Autodesk Inventor part; units mm, degrees
ref_plane "YZ Plane" through (0, 0, 0) normal (1, 0, 0) x (0, 1, 0)
ref_plane "XZ Plane" through (0, 0, 0) normal (0, 1, 0) x (-1, 0, 0)
ref_plane "XY Plane" through (0, 0, 0) normal (0, 0, 1) x (1, 0, 0)
sketch "Sketch1" plane through (0, 0, 0) normal (0, 0, 1) x (1, 0, 0)
  line L0 (0, 0) -> (40.6, 0)
  line L1 (40.6, 0) -> (40.6, 36)
  line L2 (40.6, 36) -> (0, 36)
  line L3 (0, 36) -> (0, 0)
  line L4 (0, 29) -> (-7.5, 29)
  line L5 (-7.5, 29) -> (-7.5, 26.5)
  line L6 (-7.5, 26.5) -> (0, 26.5)
  line L7 (0, 26.5) -> (0, 29)
  line L8 (40.6, 29) -> (48.1, 29)
  line L9 (48.1, 29) -> (48.1, 26.5)
  line L10 (48.1, 26.5) -> (40.6, 26.5)
  line L11 (40.6, 26.5) -> (40.6, 29)
  line L12 (0, 5) -> (-3, 5)
  line L13 (-3, 5) -> (-3, 1)
  line L14 (-3, 1) -> (0, 1)
  line L15 (0, 1) -> (0, 5)
  dimension "d0" = 40.6
  dimension "d1" = 36
  dimension "d2" = 7.5
  dimension "d3" = 2.5
  dimension "d4" = 7
  dimension "d5" = 3
  dimension "d6" = 4
  dimension "d7" = 1
extrude "Extrusion1" add sketch "Sketch1" along normal mid plane 20.3 contours L3 L2 L1 L0
extrude "Extrusion2" add sketch "Sketch1" along normal mid plane 18 contours L1 L8 L9 L10 | L6 L5 L4 L3
extrude "Extrusion3" add sketch "Sketch1" along normal mid plane 6 contours L14 L13 L12 L3
sketch "Sketch2" plane through (-7.5, 29, 9) normal (0, 1, 0) x (1, 0, 0)
  line L0 (0, 18) -> (0, 0)
  line L1 (7.5, 18) -> (7.5, 0)
  line L2 (48.1, 0) -> (48.1, 18)
  line L3 (55.6, 0) -> (48.1, 0)
  line L4 (55.6, 18) -> (55.6, 0)
  line L5 (48.1, 18) -> (55.6, 18)
  line L6 (3.5, 14) -> (3.5, 4) construction
  line L7 (0, 9) -> (55.6, 9) construction
  line L8 (52.1, 14) -> (52.1, 4) construction
  line L9 (3.5, 4) -> (52.1, 4) construction
  line L10 (52.1, 14) -> (3.5, 14) construction
  point P0 (7.5, 9)
  dimension "d14" = 3.5
  dimension "d15" = 3.5
  dimension "d16" = 10
hole "Hole1" at (-4, 29, -5) at (-4, 29, 5) at (44.6, 29, 5) at (44.6, 29, -5) direction (0, -1, 0) diameter 4 end through all
sketch "Sketch3" plane through (0, 36, 10.15) normal (0, 1, 0) x (1, 0, 0)
  line L0 (40.6, 20.3) -> (40.6, 0)
  line L1 (0, 20.3) -> (40.6, 20.3)
  circle A0 centre (30.6, 10.15) radius 7
  line L2 (0, 10.15) -> (30.6, 10.15) construction
  circle A1 centre (30.6, 10.15) radius 3
  dimension "d24" = 10
  dimension "d25" = 14
  dimension "d26" = 6
extrude "Extrusion4" add sketch "Sketch3" along normal blind 2
extrude "Extrusion5" add sketch "Sketch3" along normal blind 6 contours A1
chamfer "Chamfer1" distance 2 angle 45 1 edges at (23.6, 38, 0)
properties part number "servo HK15138"
CAD build for the part. Positions are in the model's coordinates, mm. A direction names the side the tool comes from. Coordinates: 2 decimals unless noted, no trailing zeros. Loops run counter-clockwise (first coordinate to the right, second up) from the corner with the lowest first, then second, coordinate; pieces in that order, holes last. Notation, with made-up numbers: (-31, -24.75) - (-4, -24.75) arc R24 cw to (-4, 1.25) - close; hole circle Ø3 at (-22.75, 65). An arc over 180 degrees is marked (long way). Use one line per item in the form item = value. Start each with the question number.
1) Two-plate mould, pull along Y, no slides. Class faces 1 (the face through (0, 18, 0)), 2 (the face through (26.53, 37.87, -3.12)), 3 (the face through (-4, 28, 9)): +Y half, -Y half, draft (parallel to the pull), parting line (faces both ways), or undercut.
2) Drill centre lines: L1, parallel to X at y = 28.2, z = 5; L2, parallel to Z at x = -4, y = 27.9; L3, parallel to Z at x = 44, y = 28. Where is each one in solid material? Low to high. Write a range as from..to.
3) Band-saw the part on D-D (z = 4). State how many separate pieces and enclosed holes the cut face has, and give its area (3 significant figures).
4) Band-saw the part on A-A (x = -4). Give the cut face in (y, z).
5) Band-saw the part on C-C (y = 4). Give the cut face in (x, z), and give its area (3 significant figures).
6) Tool access for faces 4 (the face through (-2, 1, 0)), 5 (the face through (33.46, 39.97, 0.9)), 6 (the face through (44, 29, 0)): list every direction of +Z, -Z, +X, -X, +Y, -Y with a clear straight run to the whole face (end or side of a thin tool).
7) Flat gauge pins, fed straight in: pin 1 (2 mm diameter, centred on y = 18, z = 1.5, fed in from -X); pin 2 (3 mm diameter, centred on y = 4, z = 0, fed in from -X); pin 3 (1.2 mm diameter, centred on x = 42.5, y = 27.5, fed in from -Z); pin 4 (12 mm diameter, centred on x = 6.5, z = -5, fed in from -Y). Where does each tip first touch, or does it go through?
Check values:
q1.face_1 = undercut
q1.face_2 = +Y half
q1.face_3 = draft
q2.L1 = -7.5..-6, -2..42.6, 46.6..48.1
q2.L2 = -9..-7, -3..3, 7..9
q2.L3 = -9..-6.91, -3.09..3.09, 6.91..9
q3.separate_pieces = 3
q3.enclosed_holes = 0
q3.area = 1,500 mm2
q4.outline = (26.5, -9) - (29, -9) - (29, -7) - (26.5, -7) - close; (26.5, -3) - (29, -3) - (29, 3) - (26.5, 3) - close; (26.5, 7) - (29, 7) - (29, 9) - (26.5, 9) - close
q5.outline = (-3, -3) - (0, -3) - (0, -10.15) - (40.6, -10.15) - (40.6, 10.15) - (0, 10.15) - (0, 3) - (-3, 3) - close
q5.area = 842 mm2
q6.face_4 = +Z, -Z, -X, -Y
q6.face_5 = +Y
q6.face_6 = +Z, -Z, +X, +Y
q7.pin_1 = 0
q7.pin_2 = -3
q7.pin_3 = -9
q7.pin_4 = 0
